from build123d import *

# Parameters (mm, degrees)
SKETCH1_R               = 3.25
BOSS_EXTRUDE1_DEPTH     = 50
CHAMFER4_SIZE           = 7
CHAMFER4_SIZE2          = 10
SKETCH2_R               = 5.5
CUT_EXTRUDE1_DEPTH      = 45
CUT_EXTRUDE3_DEPTH      = 56.397262251
CUT_EXTRUDE3_DEPTH_BACK = 50
CUT_EXTRUDE4_DEPTH      = 45
CHAMFER5_SIZE           = 5
FILLET1_R               = 3
SKETCH6_R               = 5.5
SKETCH6_R_2             = 3.25
BOSS_EXTRUDE2_DEPTH     = 11
SKETCH9_W               = 7
SKETCH9_H               = 2.5
CUT_EXTRUDE5_DEPTH      = 15


with BuildPart() as part:
    # Sketch1 → Boss-Extrude1 (new body)
    with BuildSketch(Plane(origin=(0, 0, 0), x_dir=(1, 0, 0), z_dir=(0, 1, 0))):
        Polygon((-5.320759509, 8), (-22.469015665, -7.56), (22.469015665, -7.56), (5.320759509, 8), align=None)
        with Locations(Location((0, 0, 0), (0, 0, 270))):
            Circle(SKETCH1_R, mode=Mode.SUBTRACT)
    extrude(amount=BOSS_EXTRUDE1_DEPTH)

    # Chamfer4
    chamfer4_edges = [part.edges().sort_by_distance(p)[0] for p in [
        (22.469015665, 25, 7.56),
    ]]
    chamfer4_side = [part.faces().sort_by_distance(p)[0] for p in [
        (0, 25, 7.56),
    ]]
    chamfer(chamfer4_edges, length=CHAMFER4_SIZE, length2=CHAMFER4_SIZE2, reference=chamfer4_side[0])

    # Sketch2 → Cut-Extrude1 (cut)
    with BuildSketch(Plane(origin=(0, 50, 0), x_dir=(1, 0, 0), z_dir=(0, 1, 0))):
        with Locations(Location((0, 0, 0), (0, 0, 270))):
            Circle(SKETCH2_R)
    extrude(amount=-CUT_EXTRUDE1_DEPTH, mode=Mode.SUBTRACT)

    # Sketch4 → Cut-Extrude3 (cut, two sides: drawn at the far end of the back side and taken through both)
    with BuildSketch(Plane.XZ.offset(-CUT_EXTRUDE3_DEPTH_BACK)):
        with BuildLine():
            Line((-6.5, 0), (-6.5, 8.455296228))
            Line((-6.5, 8.455296228), (-18.092934759, 18.509530088))
            Line((-18.092934759, 18.509530088), (-27.843988074, 13.266508324))
            Line((-27.843988074, 13.266508324), (-26.239796982, -3.957148404))
            Line((-26.239796982, -3.957148404), (-22.051551969, -11.746511534))
            Line((-22.051551969, -11.746511534), (6.44529607, -11.904202977))
            Line((6.44529607, -11.904202977), (12.131507072, -6.5))
            Line((12.131507072, -6.5), (0, -6.5))
            ThreePointArc((0, -6.5), (-4.596194078, -4.596194078), (-6.5, 0))
        make_face()
    extrude(amount=CUT_EXTRUDE3_DEPTH + CUT_EXTRUDE3_DEPTH_BACK, mode=Mode.SUBTRACT)

    # Sketch5 → Cut-Extrude4 (cut)
    with BuildSketch(Plane(origin=(0, 50, 0), x_dir=(1, 0, 0), z_dir=(0, 1, 0))):
        Polygon((0, 0), (4.867894822, -2.56), (20.482845708, -2.56), (8.2569175, 8.380042473), (1.341376292, 8.380042473), (-9.589048862, 8.380042473), (-9.589048862, -2.56), (-4.867894822, -2.56), align=None)
    extrude(amount=-CUT_EXTRUDE4_DEPTH, mode=Mode.SUBTRACT)

    # Chamfer5
    chamfer5_edges = [part.edges().sort_by_distance(p)[0] for p in [
        (10.017520214, 5, 2.56),
        (-5.683947411, 5, 2.56),
    ]]
    chamfer(chamfer5_edges, length=CHAMFER5_SIZE)

    # Fillet1
    fillet1_edges = [part.edges().sort_by_distance(p)[0] for p in [
        (15.318080635, 50, 5.06),
        (-6.5, 50, 5.06),
    ]]
    fillet(fillet1_edges, radius=FILLET1_R)

    # Sketch6 → Boss-Extrude2 (add)
    with BuildSketch(Plane(origin=(0, 5, 0), x_dir=(1, 0, 0), z_dir=(0, 1, 0))):
        Circle(SKETCH6_R)
        with Locations(Location((0, 0, 0), (0, 0, 270))):
            Circle(SKETCH6_R_2, mode=Mode.SUBTRACT)
    extrude(amount=BOSS_EXTRUDE2_DEPTH)

    # Sketch9 → Cut-Extrude5 (cut)
    with BuildSketch(Plane.XY.offset(7.56)):
        with Locations((4.867894822, 40)):
            Rectangle(SKETCH9_W, SKETCH9_H)
        with Locations((4.867894822, 20)):
            Rectangle(SKETCH9_W, SKETCH9_H)
    extrude(amount=-CUT_EXTRUDE5_DEPTH, mode=Mode.SUBTRACT)


solid = part.part
Could you check a few things on this model? Use its own coordinates, in mm. A direction names the side the tool comes from. Give positions to 0.01 mm unless a question says otherwise; leave off trailing zeros. Order: outer loops, then holes, each group sorted by start corner. A loop starts at its lowest first (then second) coordinate and runs counter-clockwise, first axis right, second up. Notation, with made-up numbers: (25.5, -31) - (82.5, -31) arc R18 ccw to (82.5, -2) - close; hole circle Ø9 at (-14, 36.25). An arc over 180 degrees is marked (long way). Return JSON: item names as keys, results as strings. Group by question number.
Q1. Suppose I cut it at A-A, the plane y = 11.5. Please give me the cut outline in (x, z), and give its area (3 significant figures).
Q2. Will these pins go through, and if not, where does the flat tip stop? pin 1 Ø8 at (y, z) = (34, -0.5) entering from +X; pin 2 Ø5 at (x, y) = (9.5, 37) entering from -Z; pin 3 Ø1.8 at (y, z) = (39.5, 6.5) entering from +X.
Q3. Suppose I cut it at C-C, the plane z = -0.75. Please give me the cut outline in (x, y), and give its area (3 significant figures).
Q4. Thinking about a two-plate mould opening in X: for faces 1 (the face through (6, 50, 6)), 2 (the face through (6, 41.25, 6)), 3 (the face through (14.41, 49.145, 4.988)), 4 (the face through (6, 21.25, 6)), which applies, pulls with the +X half, pulls with the -X half, needs draft (parallel to the pull), parting line crosses it, or undercut?
Q5. Suppose I cut it at D-D, the plane y = 37. Please give me the cut outline in (x, z).
Q6. Please list where these lines run through material, in increasing order: line 1 along Y through (x, z) = (6, 4); line 2 along X through (y, z) = (9.25, 0); line 3 along Z through (x, y) = (6, 35). Write a range as [from, to].
Q7. Suppose I cut it at B-B, the plane x = -0.5. Please give me the cut outline in (y, z).
Q8. Which directions (+Z, -Z, +X, -X, +Y, -Y) give clear straight access to the entire face, cutting with the end or side of a thin tool? Please do faces 5 (the face through (-0.1, 33.2, 5.5)), 6 (the face through (6, 38.75, 6)), 7 (the face through (-6.5, 24, 5)).
Resolved:
{
 "1": {"outline": "(-6.5, 2.56) - (-4.87, 2.56) arc R5.5 ccw (long way) to (4.87, 2.56) - (15.17, 2.56) - (15.47, 7.56) - (-6.5, 7.56) - close; hole circle Ø6.5 at (0, 0)", "area": "151 mm2"},
 "2": {"pin 1": "stops at x = 15.22", "pin 2": "stops at z = 2.56", "pin 3": "stops at x = 15.46"},
 "3": {"outline": "(-6.46, 0) - (-3.16, 0) - (-3.16, 16) - (-5.45, 16) - (-5.45, 6.69) - (-6.46, 6.69) - close; (3.16, 0) - (13.31, 0) - (13.31, 6.69) - (5.45, 6.69) - (5.45, 16) - (3.16, 16) - close", "area": "133 mm2"},
 "4": {"face 1": "needs draft", "face 2": "undercut", "face 3": "pulls with the +X half", "face 4": "undercut"},
 "5": {"outline": "(-6.5, 2.56) - (-4.87, 2.56) arc R5.5 cw to (4.87, 2.56) - (15.17, 2.56) - (15.47, 7.56) - (-6.5, 7.56) - close"},
 "6": {"line 1": "y = [0, 18.75], [21.25, 38.75], [41.25, 50]", "line 2": "x = [-5.5, -3.25], [3.25, 5.5]", "line 3": "z = [2.56, 7.56]"},
 "7": {"outline": "(0, -6.48) - (5, -6.48) - (5, -5.48) - (16, -5.48) - (16, -3.21) - (0, -3.21) - close; (0, 3.21) - (16, 3.21) - (16, 5.48) - (50, 5.48) - (50, 7.56) - (0, 7.56) - close"},
 "8": {"face 5": "-Z, +Y", "face 6": "+Z, -Z", "face 7": "+Z, -Z, -X, +Y, -Y"}
}
